Build history of the part. All positions in model axes, mm. Face numbers are marked on the shaded views. A direction names the side the tool comes from. Round coordinates to 2 decimals unless told otherwise and drop trailing zeros. Order: outer loops, then holes, each group sorted by start corner. A loop starts at its lowest first (then second) coordinate and runs counter-clockwise, first axis right, second up. Notation, with made-up numbers: (83.25, -14.5) -> (139.25, -14.5) arc R16 cw to (139.25, -1.5) -> close; hole circle Ø7 at (21, 37). An arc over 180 degrees is marked (long way). Use a Markdown table: item, result. Add a question column.
Item 1: Probe L1, parallel to X at y = 15, z = 0; L2, parallel to Y at x = 1, z = 3 (3 decimals). List the from-to ranges inside material, lowest first.
Item 2: Two-plate mould, pull along Z, no slides. Class the marked faces 3, 4 and 5: released by +Z, released by -Z, zero draft, split by the parting line, or undercut.
Item 3: 3-axis set-ups, long thin cutter, end or side, ignore diameter. For the marked faces 1 and 2: which of +Z, -Z, +X, -X, +Y, -Y reach the whole face in a straight line?
Item 4: Pin check, flat tips, straight feed: pin 1 (3 mm diameter, centred on y = 3.5, z = 10, fed in from +X); pin 2 (8 mm diameter, centred on x = 13.5, y = 11, fed in from -Z); pin 3 (2 mm diameter, centred on x = -11, z = -13.5, fed in from +Y). Stop position of each tip, or through.
Item 5: Slice it at A-A, the plane y = 12.25. Give the cut face in (x, z), plus the area to 3 significant figures.
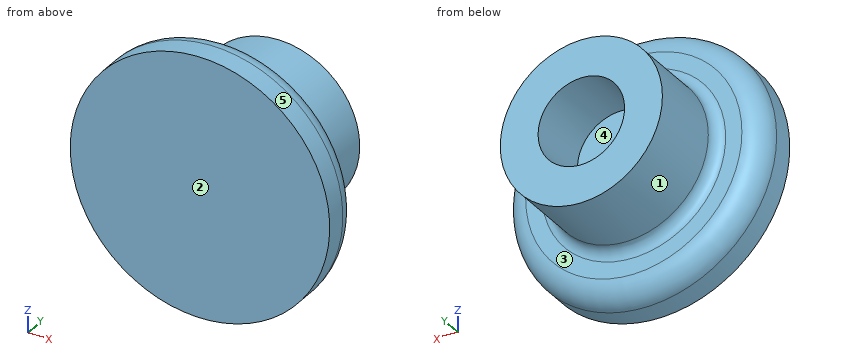
Autodesk Inventor part; units mm, degrees
ref_plane "YZ Plane" through (0, 0, 0) normal (1, 0, 0) x (0, 1, 0)
ref_plane "XZ Plane" through (0, 0, 0) normal (0, 1, 0) x (-1, 0, 0)
ref_plane "XY Plane" through (0, 0, 0) normal (0, 0, 1) x (1, 0, 0)
sketch "Sketch1" plane through (0, 0, 0) normal (0, 1, 0) x (-1, 0, 0)
  circle A0 centre (0, 0) radius 19.05
  dimension "d0" = 38.1
extrude "Extrusion1" add sketch "Sketch1" along normal blind 6.35
sketch "Sketch2" plane through (0, 6.35, 0) normal (0, 1, 0) x (1, 0, 0)
  circle A0 centre (0, 0) radius 11.9062
  dimension "d3" = 23.8125
extrude "Extrusion2" add sketch "Sketch2" along normal blind 12.7
sketch "Sketch3" plane through (0, 19.05, 0) normal (0, 1, 0) x (1, 0, 0)
  circle A0 centre (0, 0) radius 11.9062
hole "Hole1" at (0, 19.05, 0) direction (0, -1, 0) diameter 12.7 depth 9.525
fillet "Fillet1" radius 1.5875 1 edges at (-11.9062, 6.35, 0)
fillet "Fillet2" radius 3.175 1 edges at (19.05, 6.35, 0)
properties part number "Feet"
Check sheet entries:
| question | item | result |
|---|---|---|
| 1 | L1 | -11.91 to -6.35, 6.35 to 11.91 |
| 1 | L2 | 0 to 9.525 |
| 2 | face 3 | zero draft |
| 2 | face 4 | undercut |
| 2 | face 5 | split by the parting line |
| 3 | face 1 | +Y |
| 3 | face 2 | +Z, -Z, +X, -X, -Y |
| 4 | pin 1 | x = 17.04 |
| 4 | pin 2 | z = -7.18 |
| 4 | pin 3 | y = 6.3 |
| 5 | outline | circle Ø23.81 at (0, 0); hole circle Ø12.7 at (0, 0) |
| 5 | area | 319 mm2 |
